Geometry: see drawing. Coordinates: mm, zero at the bounding-box minimum. Give positions to 0.01 mm unless a question says otherwise; leave off trailing zeros. Order: outer loops, then holes, each group sorted by start corner. A loop starts at its lowest first (then second) coordinate and runs counter-clockwise, first axis right, second up. Notation, with made-up numbers: (71.25, -24.5) - (113.25, -24.5) arc R17 ccw to (113.25, -2.5) - close; hole circle Ø1 at (83, -21). An arc over 180 degrees is marked (long way). Put each result on its own line as item: value. Start each with the question number.
1. Ray query, line 1 along X through (y, z) = (0.65, 5); line 2 along Z through (x, y) = (4.5, 0.25); line 3 along X through (y, z) = (0.5, 6.5). Return the intervals inside material, ascending. Write a range as from..to.
2. Section A-A on z = 5. Return the cut outline in (x, y).
3. Section D-D on x = 24.75. Return the cut outline in (y, z).
4. Section C-C on y = 0.7. Return the cut outline in (x, z).
5. Section B-B on x = 4.5. Return the cut outline in (y, z), plus the area to 3 significant figures.
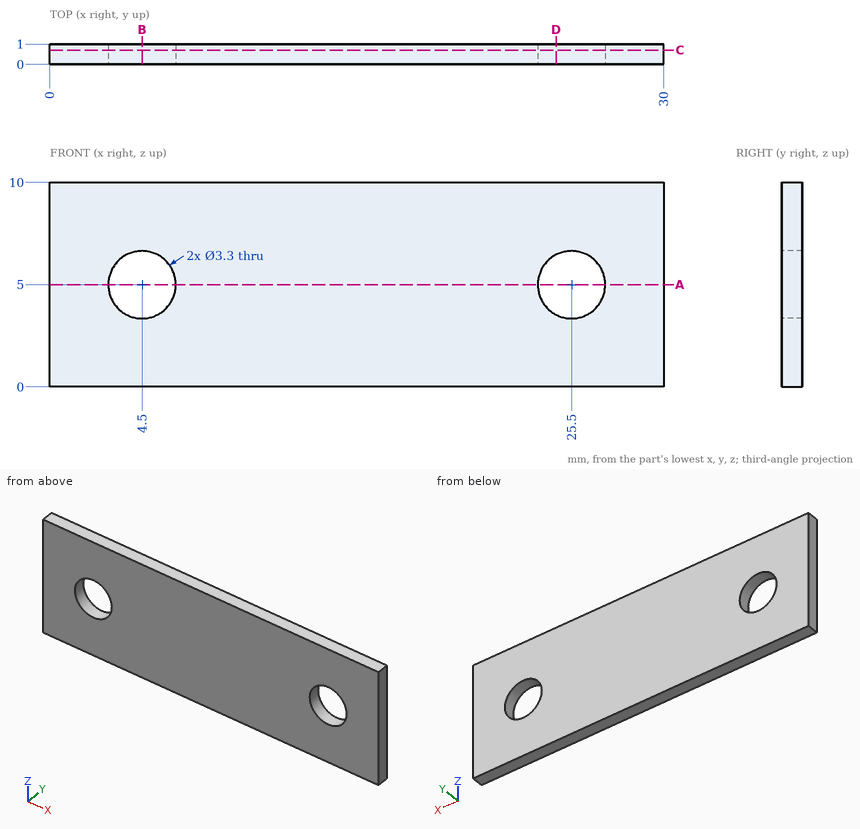
Resolved:
1. line 1: 0..2.85, 6.15..23.85, 27.15..30
1. line 2: 0..3.35, 6.65..10
1. line 3: 0..3.81, 5.19..24.81, 26.19..30
2. outline: (0, 0) - (2.85, 0) - (2.85, 1) - (0, 1) - close; (6.15, 0) - (23.85, 0) - (23.85, 1) - (6.15, 1) - close; (27.15, 0) - (30, 0) - (30, 1) - (27.15, 1) - close
3. outline: (0, 0) - (1, 0) - (1, 3.53) - (0, 3.53) - close; (0, 6.47) - (1, 6.47) - (1, 10) - (0, 10) - close
4. outline: (0, 0) - (30, 0) - (30, 10) - (0, 10) - close; hole circle Ø3.3 at (4.5, 5); hole circle Ø3.3 at (25.5, 5)
5. outline: (0, 0) - (1, 0) - (1, 3.35) - (0, 3.35) - close; (0, 6.65) - (1, 6.65) - (1, 10) - (0, 10) - close
5. area: 6.70 mm^2
